Geometry: final body of the model. Coordinates: model frame, mm. Face numbers are marked on the shaded views. Give positions to 0.01 mm unless a question says otherwise; leave off trailing zeros. Write each loop counter-clockwise with the first axis right and the second up, starting at its lowest first coordinate (ties: lowest second). Pieces come first, ordered by that corner, then holes.
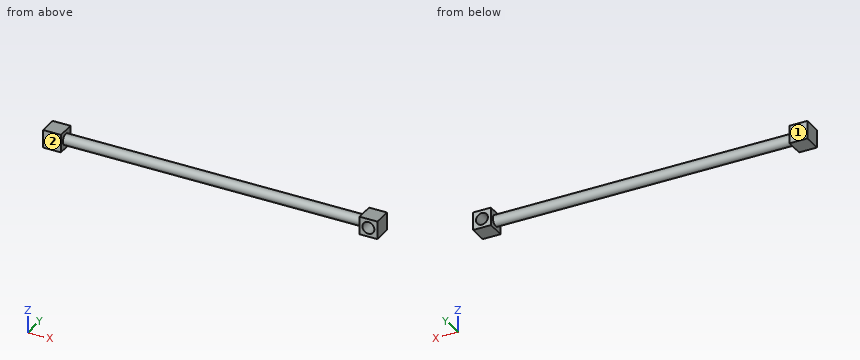
from build123d import *

# Parameters (mm, degrees)
SKETCH1_W           = 30
SKETCH1_H           = 30
BOSS_EXTRUDE1_DEPTH = 30
SKETCH2_R           = 9
BOSS_EXTRUDE2_DEPTH = 500
SKETCH3_W           = 30
SKETCH3_H           = 30
BOSS_EXTRUDE3_DEPTH = 30
SKETCH4_R           = 10
CUT_EXTRUDE1_DEPTH  = 30


with BuildPart() as part:
    # Sketch1 → Boss-Extrude1 (new body)
    with BuildSketch(Plane(origin=(0, 0, 0), x_dir=(0, 0, -1), z_dir=(1, 0, 0))):
        Rectangle(SKETCH1_W, SKETCH1_H)
    extrude(amount=BOSS_EXTRUDE1_DEPTH)

    # Sketch2 → Boss-Extrude2 (add)
    with BuildSketch(Plane(origin=(30, 0, 0), x_dir=(0, 0, -1), z_dir=(1, 0, 0))):
        Circle(SKETCH2_R)
    extrude(amount=BOSS_EXTRUDE2_DEPTH)

    # Sketch3 → Boss-Extrude3 (add)
    with BuildSketch(Plane(origin=(530, 0, 0), x_dir=(0, 0, -1), z_dir=(1, 0, 0))):
        Rectangle(SKETCH3_W, SKETCH3_H)
    extrude(amount=BOSS_EXTRUDE3_DEPTH)

    # Sketch4 → Cut-Extrude1 (cut)
    with BuildSketch(Plane(origin=(0, 15, 0), x_dir=(1, 0, 0), z_dir=(0, 1, 0))):
        with Locations((545, 0)):
            Circle(SKETCH4_R)
    extrude(amount=-CUT_EXTRUDE1_DEPTH, mode=Mode.SUBTRACT)


solid = part.part
Q1. Section B-B on x = 545. Output: boundary loops of the cut face in (y, z).
Filled sheet:
outline: (-15, -15) - (15, -15) - (15, -10) - (-15, -10) - close; (-15, 10) - (15, 10) - (15, 15) - (-15, 15) - close
Q2. Section A-A on z = 0. Output: boundary loops of the cut face in (x, y).
Filled sheet:
outline: (0, -15) - (30, -15) - (30, -9) - (530, -9) - (530, -15) - (535, -15) - (535, 15) - (530, 15) - (530, 9) - (30, 9) - (30, 15) - (0, 15) - close; (555, -15) - (560, -15) - (560, 15) - (555, 15) - close
Q3. Ray query, line 1 along X through (y, z) = (-3, 0); line 2 along Z through (x, y) = (545, -0.25); line 3 along X through (y, z) = (-11.5, -11.5). Return the intervals inside material, ascending.
Filled sheet:
line 1: x = 0 to 535, 555 to 560
line 2: z = -15 to -10, 10 to 15
line 3: x = 0 to 30, 530 to 560
Q4. Pull-direction query (Y, two-part tool) for the marked faces 1 and 2; classes: released by +Y, released by -Y, zero draft, split by the parting line, or undercut.
Filled sheet:
face 1: released by +Y
face 2: released by -Y
Q5. Section D-D on x = 406. Output: boundary loops of the cut face in (y, z).
Filled sheet:
outline: circle Ø18 at (0, 0)
Q6. Pin query (flat end, axial travel): P1, Ø10, axis at x = 414, y = 10.5, coming from the +Z side; P2, Ø6, axis at x = 343.5, z = -1.5, coming from the +Y side; P3, Ø3, axis at x = 101, y = 11.5, coming from the +Z side; P4, Ø4, axis at x = 298, y = -2, coming from the +Z side. Return the tip coordinate at first contact, or that it passes through.
Filled sheet:
P1: stops at z = 7.12
P2: stops at y = 9
P3: passes through
P4: stops at z = 9
Q7. Section C-C on y = 0. Output: boundary loops of the cut face in (x, z), plus the area to 3 significant figures.
Filled sheet:
outline: (0, -15) - (30, -15) - (30, -9) - (530, -9) - (530, -15) - (560, -15) - (560, 15) - (530, 15) - (530, 9) - (30, 9) - (30, 15) - (0, 15) - close; hole circle Ø20 at (545, 0)
area: 10,500 mm2
